Here's how the part is built. I have some questions about the finished solid (model axes, mm). A direction names the side the tool comes from. Coordinates: 2 decimals unless noted, no trailing zeros. Order: outer loops, then holes, each group sorted by start corner. A loop starts at its lowest first (then second) coordinate and runs counter-clockwise, first axis right, second up. Notation, with made-up numbers: (13, -5.5) -> (23, -5.5) arc R16 ccw to (23, 18.5) -> close; hole circle Ø2 at (17, 35). An arc over 180 degrees is marked (long way). One line per item, written item: value. Start each with the question number.
```python
from build123d import *

# Parameters (mm, degrees)
FLANGE_BASE2_DEPTH         = 1517.3
ESBO_O10_R                 = 15
ESBO_O10_R_2               = 2.1
ESBO_O10_R_3               = 3.4
ESBO_O10_W                 = 100
ESBO_O10_H                 = 210.6
ESBO_O10_H_2               = 150
CORTE_EXTRUS_O1_DEPTH      = 1532.196117452
CORTE_EXTRUS_O2_DEPTH      = 1543.569660534
CORTE_EXTRUS_O2_DEPTH_BACK = 1543.569660534
CORTE_EXTRUS_O3_DEPTH      = 1543.569660534
CORTE_EXTRUS_O3_DEPTH_BACK = 10
ESBO_O12_R                 = 15


# Sheet-metal steps are written as plain solids
with BuildPart() as part:
    # Esboço1 → Flange-base2 (new body)
    with BuildSketch(Plane.XY):
        with BuildLine():
            Line((-107.95, -175.24), (-107.95, -13.35))
            ThreePointArc((-107.95, -13.35), (-104.039875529, -3.910124471), (-94.6, 0))
            Line((-94.6, 0), (94.6, 0))
            ThreePointArc((94.6, 0), (104.039875529, -3.910124471), (107.95, -13.35))
            Line((107.95, -13.35), (107.95, -175.24))
            Line((107.95, -175.24), (101.6, -175.24))
            Line((101.6, -175.24), (101.6, -13.35))
            ThreePointArc((101.6, -13.35), (99.549747468, -8.400252532), (94.6, -6.35))
            Line((94.6, -6.35), (-94.6, -6.35))
            ThreePointArc((-94.6, -6.35), (-99.549747468, -8.400252532), (-101.6, -13.35))
            Line((-101.6, -13.35), (-101.6, -175.24))
            Line((-101.6, -175.24), (-107.95, -175.24))
        make_face()
    extrude(amount=-FLANGE_BASE2_DEPTH)

    # Esboço10 → Corte-extrusão1 (cut, through all)
    with BuildSketch(Plane(origin=(0, 0, 0), x_dir=(1, 0, 0), z_dir=(0, 1, 0))):
        with Locations(Location((0, 1452.3, 0), (0, 0, 270))):
            Circle(ESBO_O10_R)
        with Locations(Location((-20, 1452.3, 0), (0, 0, 270))):
            Circle(ESBO_O10_R_2)
        with Locations(Location((10, 1469.620508076, 0), (0, 0, 270))):
            Circle(ESBO_O10_R_2)
        with Locations(Location((10, 1434.979491924, 0), (0, 0, 270))):
            Circle(ESBO_O10_R_2)
        with Locations(Location((-60.6, 1365.7, 0), (0, 0, 270))):
            Circle(ESBO_O10_R_3)
        with Locations(Location((60.6, 1365.7, 0), (0, 0, 270))):
            Circle(ESBO_O10_R_3)
        with Locations(Location((60.6, 1133.9, 0), (0, 0, 270))):
            Circle(ESBO_O10_R_3)
        with Locations(Location((-60.6, 1133.9, 0), (0, 0, 270))):
            Circle(ESBO_O10_R_3)
        with Locations(Location((-20.2, 1365.7, 0), (0, 0, 270))):
            Circle(ESBO_O10_R_3)
        with Locations(Location((20.2, 1365.7, 0), (0, 0, 270))):
            Circle(ESBO_O10_R_3)
        with Locations(Location((-60.6, 1191.85, 0), (0, 0, 270))):
            Circle(ESBO_O10_R_3)
        with Locations(Location((-60.6, 1249.8, 0), (0, 0, 270))):
            Circle(ESBO_O10_R_3)
        with Locations(Location((-60.6, 1307.75, 0), (0, 0, 270))):
            Circle(ESBO_O10_R_3)
        with Locations(Location((20.2, 1133.9, 0), (0, 0, 270))):
            Circle(ESBO_O10_R_3)
        with Locations(Location((-20.2, 1133.9, 0), (0, 0, 270))):
            Circle(ESBO_O10_R_3)
        with Locations(Location((60.6, 1191.85, 0), (0, 0, 270))):
            Circle(ESBO_O10_R_3)
        with Locations(Location((60.6, 1249.8, 0), (0, 0, 270))):
            Circle(ESBO_O10_R_3)
        with Locations(Location((60.6, 1307.75, 0), (0, 0, 270))):
            Circle(ESBO_O10_R_3)
        with Locations(Location((-60.6, 853.1, 0), (0, 0, 270))):
            Circle(ESBO_O10_R_3)
        with Locations(Location((60.6, 853.1, 0), (0, 0, 270))):
            Circle(ESBO_O10_R_3)
        with Locations(Location((60.6, 681.9, 0), (0, 0, 270))):
            Circle(ESBO_O10_R_3)
        with Locations(Location((-60.6, 681.9, 0), (0, 0, 270))):
            Circle(ESBO_O10_R_3)
        with Locations(Location((-20.2, 853.1, 0), (0, 0, 270))):
            Circle(ESBO_O10_R_3)
        with Locations(Location((20.2, 853.1, 0), (0, 0, 270))):
            Circle(ESBO_O10_R_3)
        with Locations(Location((-60.6, 738.966666667, 0), (0, 0, 270))):
            Circle(ESBO_O10_R_3)
        with Locations(Location((-60.6, 796.033333333, 0), (0, 0, 270))):
            Circle(ESBO_O10_R_3)
        with Locations(Location((20.2, 681.9, 0), (0, 0, 270))):
            Circle(ESBO_O10_R_3)
        with Locations(Location((-20.2, 681.9, 0), (0, 0, 270))):
            Circle(ESBO_O10_R_3)
        with Locations(Location((60.6, 738.966666667, 0), (0, 0, 270))):
            Circle(ESBO_O10_R_3)
        with Locations(Location((60.6, 796.033333333, 0), (0, 0, 270))):
            Circle(ESBO_O10_R_3)
        with Locations((0, 1249.8)):
            Rectangle(ESBO_O10_W, ESBO_O10_H)
        with Locations((0, 767.5)):
            Rectangle(ESBO_O10_W, ESBO_O10_H_2)
        with BuildLine():
            Line((-20, 20), (-20, 0))
            Line((-20, 0), (20, 0))
            Line((20, 0), (20, 20))
            ThreePointArc((20, 20), (0, 40), (-20, 20))
        make_face()
    extrude(amount=-CORTE_EXTRUS_O1_DEPTH, mode=Mode.SUBTRACT)

    # Esboço11 → Corte-extrusão2 (cut, two sides: drawn at the far end of the back side and taken through both)
    with BuildSketch(Plane(origin=(107.95, 0, 0), x_dir=(0, 0, -1), z_dir=(1, 0, 0)).offset(-CORTE_EXTRUS_O2_DEPTH_BACK)):
        with BuildLine():
            Line((161.89, -175.24), (267.89, -175.24))
            Line((267.89, -175.24), (267.89, -84.54))
            ThreePointArc((267.89, -84.54), (263.789494937, -74.640505063), (253.89, -70.54))
            Line((253.89, -70.54), (175.89, -70.54))
            ThreePointArc((175.89, -70.54), (165.990505063, -74.640505063), (161.89, -84.54))
            Line((161.89, -84.54), (161.89, -175.24))
        make_face()
    extrude(amount=CORTE_EXTRUS_O2_DEPTH + CORTE_EXTRUS_O2_DEPTH_BACK, mode=Mode.SUBTRACT)

    # Esboço12 → Corte-extrusão3 (cut, two sides: drawn at the far end of the back side and taken through both)
    with BuildSketch(Plane.ZY.offset(107.95).offset(-CORTE_EXTRUS_O3_DEPTH_BACK)):
        with Locations(Location((-1239.9, -128.76, 0), (0, 0, 90))):
            Circle(ESBO_O12_R)
        with Locations(Location((-691.9, -45.24, 0), (0, 0, 90))):
            Circle(ESBO_O12_R)
    extrude(amount=CORTE_EXTRUS_O3_DEPTH + CORTE_EXTRUS_O3_DEPTH_BACK, mode=Mode.SUBTRACT)


solid = part.part
```
Q1. I need wall thicknesses on line 1 (X direction, y = -2, z = -1191.85); line 2 (Z direction, x = -104, y = -128.76); line 3 (X direction, y = -2, z = -1452.3). Which ranges of each line are inside material? Lowest first, please.
Q2. Imagine slicing it at A-A (y = -160). Write out the boundary of the cut face in (x, z), plus the area to 3 significant figures.
Q3. If we mould it in two halves opening along Z, with no side actions, what happens to faces 4 (the face through (10.138, -3.131, -1463.356)), 5 (the face through (101.6, -95, -748)), 6 (the face through (103, -61, 0))? For each: +Z half, -Z half, draft (parallel to the pull), parting line (faces both ways), or undercut.
Q4. Imagine slicing it at B-B (z = -1410). Write out the boundary of the cut face in (x, y), plus the area to 3 significant figures.
Q5. For faces 1 (the face through (64, -6.35, -748)), 2 (the face through (-104.731, -132.012, -1225.257)), 3 (the face through (1, -3, -1517.3)), which set-ups out of +Z, -Z, +X, -X, +Y, -Y let a thin tool reach every point of the face, with its end or its side?
Q6. For P1, Ø8, axis at x = -60.6, z = -1249.8, coming from the -Y side; P2, Ø1.9, axis at x = 103.5, z = -205.5, coming from the -Y side; P3, Ø18, axis at x = 0, z = -1452.3, coming from the -Y side; P4, Ø3, axis at y = -2, z = -1267.5, coming from the +X side, each with a flat end and sliding along its axis, tell me the tip position at first contact or that it passes through.
Completed:
1. line 1: x = -101.63 to -64, -57.2 to -50, 50 to 57.2, 64 to 101.63
1. line 2: z = -1517.3 to -1254.9, -1224.9 to -267.89, -161.89 to 0
1. line 3: x = -101.63 to -22.1, -17.9 to -15, 15 to 101.63
2. outline: (-107.95, -1517.3) -> (-101.6, -1517.3) -> (-101.6, -267.89) -> (-107.95, -267.89) -> close; (-107.95, -161.89) -> (-101.6, -161.89) -> (-101.6, 0) -> (-107.95, 0) -> close; (101.6, -1517.3) -> (107.95, -1517.3) -> (107.95, -267.89) -> (101.6, -267.89) -> close; (101.6, -161.89) -> (107.95, -161.89) -> (107.95, 0) -> (101.6, 0) -> close
2. area: 17,900 mm2
3. face 4: undercut
3. face 5: draft
3. face 6: +Z half
4. outline: (-107.95, -175.24) -> (-101.6, -175.24) -> (-101.6, -13.35) arc R7 cw to (-94.6, -6.35) -> (94.6, -6.35) arc R7 cw to (101.6, -13.35) -> (101.6, -175.24) -> (107.95, -175.24) -> (107.95, -13.35) arc R13.35 ccw to (94.6, 0) -> (-94.6, 0) arc R13.35 ccw to (-107.95, -13.35) -> close
4. area: 3,460 mm2
5. face 1: +Z, -Z, -Y
5. face 2: -X
5. face 3: -Z, +X, -X, +Y, -Y
6. P1: stops at y = -6.35
6. P2: stops at y = -70.54
6. P3: passes through
6. P4: stops at x = 103.61
